```python
from build123d import *

# Parameters (mm, degrees)
SKETCH1_W           = 61
SKETCH1_H           = 42
BOSS_EXTRUDE1_DEPTH = 2
SKETCH2_W           = 61
SKETCH2_H           = 42
SKETCH2_W_2         = 57
SKETCH2_H_2         = 38
BOSS_EXTRUDE2_DEPTH = 3
SKETCH3_W           = 5.775270692
SKETCH3_H           = 15
SKETCH3_W_2         = 6.454719949
SKETCH3_H_2         = 8
CUT_EXTRUDE1_DEPTH  = 5
SKETCH4_R           = 2
BOSS_EXTRUDE3_DEPTH = 2
SKETCH5_W           = 10
SKETCH5_H           = 3.5
BOSS_EXTRUDE4_DEPTH = 2
FILLET1_R           = 1
FILLET2_R           = 1


with BuildPart() as part:
    # Sketch1 → Boss-Extrude1 (new body)
    with BuildSketch(Plane(origin=(0, 0, 0), x_dir=(1, 0, 0), z_dir=(0, 1, 0))):
        with Locations((9.74023618, -1.906412613)):
            Rectangle(SKETCH1_W, SKETCH1_H)
    extrude(amount=BOSS_EXTRUDE1_DEPTH)

    # Sketch2 → Boss-Extrude2 (add)
    with BuildSketch(Plane(origin=(0, 2, 0), x_dir=(1, 0, 0), z_dir=(0, 1, 0))):
        with Locations((9.74023618, -1.906412613)):
            Rectangle(SKETCH2_W, SKETCH2_H)
        with Locations((9.74023618, -1.906412613)):
            Rectangle(SKETCH2_W_2, SKETCH2_H_2, mode=Mode.SUBTRACT)
    extrude(amount=BOSS_EXTRUDE2_DEPTH)

    # Sketch3 → Cut-Extrude1 (cut)
    with BuildSketch(Plane(origin=(0, 5, 0), x_dir=(1, 0, 0), z_dir=(0, 1, 0))):
        with Locations((-20.110444063, -1.906412613)):
            Rectangle(SKETCH3_W, SKETCH3_H)
        with Locations((38.800224202, -1.906412613)):
            Rectangle(SKETCH3_W_2, SKETCH3_H_2)
    extrude(amount=-CUT_EXTRUDE1_DEPTH, mode=Mode.SUBTRACT)

    # Sketch4 → Boss-Extrude3 (add)
    with BuildSketch(Plane(origin=(0, 2, 0), x_dir=(1, 0, 0), z_dir=(0, 1, 0))):
        with Locations((-14.25976382, -15.906412613)):
            Circle(SKETCH4_R)
        with Locations((-14.25976382, 12.093587387)):
            Circle(SKETCH4_R)
        with Locations((33.74023618, 12.093587387)):
            Circle(SKETCH4_R)
        with Locations((33.74023618, -15.906412613)):
            Circle(SKETCH4_R)
    extrude(amount=BOSS_EXTRUDE3_DEPTH)

    # Sketch5 → Boss-Extrude4 (add)
    with BuildSketch(Plane(origin=(0, 5, 0), x_dir=(1, 0, 0), z_dir=(0, 1, 0))):
        with Locations((9.74023618, -21.156412613)):
            Rectangle(SKETCH5_W, SKETCH5_H)
        with Locations((9.74023618, 17.343587387)):
            Rectangle(SKETCH5_W, SKETCH5_H)
    extrude(amount=BOSS_EXTRUDE4_DEPTH)

    # Fillet1
    fillet1_edges = [part.edges().sort_by_distance(p)[0] for p in [
        (9.74023618, 5, 20.906412613),
        (9.74023618, 5, -17.093587387),
    ]]
    fillet(fillet1_edges, radius=FILLET1_R)

    # Fillet2
    fillet2_edges = [part.edges().sort_by_distance(p)[0] for p in [
        (27.49023618, 5, 22.906412613),
        (9.74023618, 7, 22.906412613),
        (-8.00976382, 5, -19.093587387),
        (9.74023618, 7, -19.093587387),
        (-20.75976382, 5, -12.343587387),
        (-8.00976382, 5, 22.906412613),
        (40.24023618, 5, 14.406412613),
        (27.49023618, 5, -19.093587387),
        (-20.75976382, 5, 16.156412613),
        (40.24023618, 5, -10.593587387),
    ]]
    fillet(fillet2_edges, radius=FILLET2_R)


solid = part.part
```
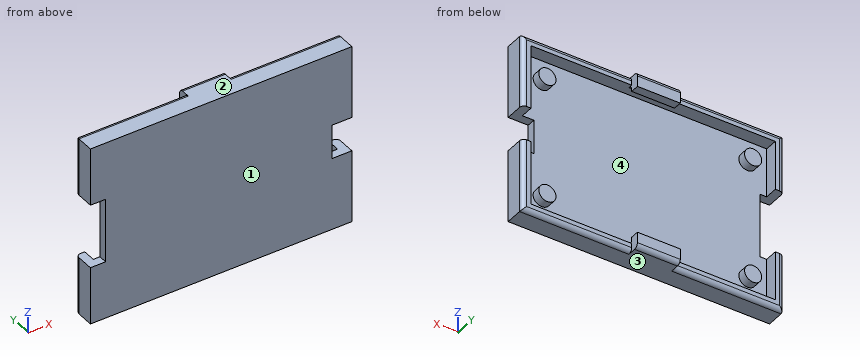
Design review of the part built by this model. Coordinates are the model's own, in mm. Face numbers are marked on the shaded views. Coordinates: 2 decimals unless noted, no trailing zeros. Write each loop counter-clockwise with the first axis right and the second up, starting at its lowest first coordinate (ties: lowest second). Pieces come first, ordered by that corner, then holes.
1) Add section C-C (x = 10). Write out the cut boundary in (y, z).
2) Add section A-A (y = 3.25). Write out the cut boundary in (x, z).
3) Mouldability with a two-part tool opening along Z and no side actions: class the marked faces 1, 2, 3 and 4 as +Z half, -Z half, draft (parallel to the pull), parting line (faces both ways), or undercut.
4) Add section B-B (z = -9). Write out the cut boundary in (x, y).
5) To check wall thickness, follow L1, parallel to X at y = 2.25, z = -9; L2, parallel to Z at x = 6.5, y = 2.75; L3, parallel to Y at x = 10, z = -8.5. State the ranges of each line that lie inside material, in increasing order.
6) Insertion check: pin 1 (10 mm diameter, centred on x = -6.5, z = 18, fed in from +Y); pin 2 (5 mm diameter, centred on x = 32, z = 11.5, fed in from +Y); pin 3 (1.2 mm diameter, centred on x = -13.5, z = -11.5, fed in from +Y). Each pin has a flat end and moves straight along its axis. Give the tip position at first contact, or say it passes through.
7) Add section D-D (x = 18). Write out the cut boundary in (y, z).
Check result:
1. outline: (0, -19.09) - (6, -19.09) arc R1 ccw to (7, -18.09) - (7, -15.59) - (5, -15.59) - (5, -16.09) arc R1 cw to (4, -17.09) - (2, -17.09) - (2, 20.91) - (4, 20.91) arc R1 cw to (5, 19.91) - (5, 19.41) - (7, 19.41) - (7, 21.91) arc R1 ccw to (6, 22.91) - (0, 22.91) - close
2. outline: (-20.76, -19.09) - (40.24, -19.09) - (40.24, -2.09) - (38.24, -2.09) - (38.24, -17.09) - (-18.76, -17.09) - (-18.76, -5.59) - (-20.76, -5.59) - close; (-20.76, 9.41) - (-18.76, 9.41) - (-18.76, 20.91) - (38.24, 20.91) - (38.24, 5.91) - (40.24, 5.91) - (40.24, 22.91) - (-20.76, 22.91) - close; circle Ø4 at (-14.26, -12.09); circle Ø4 at (-14.26, 15.91); circle Ø4 at (33.74, -12.09); circle Ø4 at (33.74, 15.91)
3. face 1: draft
3. face 2: +Z half
3. face 3: -Z half
3. face 4: undercut
4. outline: (-20.76, 0) - (40.24, 0) - (40.24, 4) arc R1 ccw to (39.24, 5) - (38.24, 5) - (38.24, 2) - (-18.76, 2) - (-18.76, 5) - (-19.76, 5) arc R1 ccw to (-20.76, 4) - close
5. L1: x = -20.76 to -18.76, 38.24 to 40.24
5. L2: z = -19.09 to -17.09, 20.91 to 22.91
5. L3: y = 0 to 2
6. pin 1: stops at y = 5
6. pin 2: stops at y = 2
6. pin 3: stops at y = 4
7. outline: (0, -19.09) - (4, -19.09) arc R1 ccw to (5, -18.09) - (5, -17.09) - (2, -17.09) - (2, 20.91) - (5, 20.91) - (5, 21.91) arc R1 ccw to (4, 22.91) - (0, 22.91) - close
